Build history of the part. All positions in model axes, mm. A direction names the side the tool comes from. Coordinates: 2 decimals unless noted, no trailing zeros. Order: outer loops, then holes, each group sorted by start corner. A loop starts at its lowest first (then second) coordinate and runs counter-clockwise, first axis right, second up. Notation, with made-up numbers: (35, 53) - (72, 53) arc R8 ccw to (72, 58) - close; hole circle Ø3 at (89.25, 51). An arc over 180 degrees is marked (long way). Write each question's results on one line, items separated by ' | '.
from build123d import *

# Parameters (mm, degrees)
SKETCH1_R               = 13
SKETCH1_R_2             = 1.6
BOSS_EXTRUDE1_DEPTH     = 6.35
SKETCH2_W               = 5.8
SKETCH2_H               = 43
BOSS_EXTRUDE2_DEPTH     = 25.4
CUT_EXTRUDE1_DEPTH      = 26.4
CUT_EXTRUDE1_DEPTH_BACK = 7.35
SKETCH5_R               = 3.571875
CUT_EXTRUDE2_DEPTH      = 49.8
CUT_EXTRUDE2_DEPTH_BACK = 6.8
CHAMFER1_SIZE           = 5


with BuildPart() as part:
    # Sketch1 → Boss-Extrude1 (new body)
    with BuildSketch(Plane.XY):
        Polygon((-21.5, 21.5), (21.5, 21.5), (27.3, 21.5), (27.3, -21.5), (21.5, -21.5), (-21.5, -21.5), (-27.3, -21.5), (-27.3, 21.5), align=None)
        Circle(SKETCH1_R, mode=Mode.SUBTRACT)
        with Locations((-15.5, 15.5)):
            Circle(SKETCH1_R_2, mode=Mode.SUBTRACT)
        with Locations((15.5, 15.5)):
            Circle(SKETCH1_R_2, mode=Mode.SUBTRACT)
        with Locations((15.5, -15.5)):
            Circle(SKETCH1_R_2, mode=Mode.SUBTRACT)
        with Locations((-15.5, -15.5)):
            Circle(SKETCH1_R_2, mode=Mode.SUBTRACT)
    extrude(amount=BOSS_EXTRUDE1_DEPTH)

    # Sketch2 → Boss-Extrude2 (add)
    with BuildSketch(Plane.XY.offset(6.35)):
        with Locations((-24.4, 0)):
            Rectangle(SKETCH2_W, SKETCH2_H)
        with Locations((24.4, 0)):
            Rectangle(SKETCH2_W, SKETCH2_H)
    extrude(amount=BOSS_EXTRUDE2_DEPTH)

    # Sketch4 → Cut-Extrude1 (cut, two sides)
    with BuildSketch(Plane.XY.offset(6.35)) as cut_extrude1_sk:
        Polygon((-27.3, 12.7), (-21.5, 12.7), (-21.5, 16.5), (-16.5, 21.5), (-21.5, 21.5), (-27.3, 21.5), align=None)
        Polygon((21.5, 21.5), (16.5, 21.5), (21.5, 16.5), (21.5, 12.7), (27.3, 12.7), (27.3, 21.5), align=None)
        Polygon((27.3, -21.5), (27.3, -12.7), (21.5, -12.7), (21.5, -16.5), (16.5, -21.5), (21.5, -21.5), align=None)
        Polygon((-27.3, -21.5), (-21.5, -21.5), (-16.5, -21.5), (-21.5, -16.5), (-21.5, -12.7), (-27.3, -12.7), align=None)
    extrude(amount=CUT_EXTRUDE1_DEPTH, mode=Mode.SUBTRACT)
    extrude(cut_extrude1_sk.sketch, amount=-CUT_EXTRUDE1_DEPTH_BACK, mode=Mode.SUBTRACT)

    # Sketch5 → Cut-Extrude2 (cut, two sides)
    with BuildSketch(Plane(origin=(-21.5, 0, 0), x_dir=(0, 0, -1), z_dir=(1, 0, 0))) as cut_extrude2_sk:
        with Locations((-19.05, 0)):
            Circle(SKETCH5_R)
    extrude(amount=CUT_EXTRUDE2_DEPTH, mode=Mode.SUBTRACT)
    extrude(cut_extrude2_sk.sketch, amount=-CUT_EXTRUDE2_DEPTH_BACK, mode=Mode.SUBTRACT)

    # Chamfer1
    chamfer1_edges = [part.edges().sort_by_distance(p)[0] for p in [
        (21.5, -12.7, 19.05),
        (-21.5, 12.7, 19.05),
        (-21.5, -12.7, 19.05),
        (21.5, 12.7, 19.05),
    ]]
    chamfer(chamfer1_edges, length=CHAMFER1_SIZE)


solid = part.part
1. Band-saw the part on A-A on z = 19.05. Give the cut face in (x, y), then the cut area to 3 significant figures.
Solved:
outline: (-27.3, -12.7) - (-26.5, -12.7) - (-21.5, -7.7) - (-21.5, -3.57) - (-27.3, -3.57) - close; (-27.3, 3.57) - (-21.5, 3.57) - (-21.5, 7.7) - (-26.5, 12.7) - (-27.3, 12.7) - close; (21.5, -7.7) - (26.5, -12.7) - (27.3, -12.7) - (27.3, -3.57) - (21.5, -3.57) - close; (21.5, 3.57) - (27.3, 3.57) - (27.3, 12.7) - (26.5, 12.7) - (21.5, 7.7) - close | area: 162 mm2
2. Drop flat-ended pins along their axis: pin 1 Ø4 at (x, y) = (15.5, -15.5) entering from +Z; pin 2 Ø4.5 at (x, z) = (25.5, 21.5) entering from +Y; pin 3 Ø4.5 at (x, z) = (-23, 11) entering from -Y; pin 4 Ø2.5 at (x, y) = (-15.5, 15.5) entering from -Z. Give the stop position or say it passes through.
Solved:
pin 1: stops at z = 6.35 | pin 2: stops at y = 12.7 | pin 3: stops at y = -11.45 | pin 4: passes through
3. Two-plate mould, pull along Y, no slides. Class faces 1 (the face through (-19, 19, 3)), 2 (the face through (-16.68, 16.58, 3.13)), 3 (the face through (24, -10.2, 18.9)), 4 (the face through (-24, 0, 31.75)): +Y half, -Y half, draft (parallel to the pull), parting line (faces both ways), or undercut.
Solved:
face 1: +Y half | face 2: undercut | face 3: -Y half | face 4: draft
4. Tool access for faces 5 (the face through (21.5, -15, 3)), 6 (the face through (-27, -12.7, 9)), 7 (the face through (21.5, -4, 22)): list every direction of +Z, -Z, +X, -X, +Y, -Y with a clear straight run to the whole face (end or side of a thin tool).
Solved:
face 5: +Z, -Z, +X, -Y | face 6: +Z, -Z, -X, -Y | face 7: +Z, +Y, -Y
5. Band-saw the part on D-D on z = 11. Give the cut face in (x, y).
Solved:
outline: (-27.3, -12.7) - (-26.5, -12.7) - (-21.5, -7.7) - (-21.5, 7.7) - (-26.5, 12.7) - (-27.3, 12.7) - close; (21.5, -7.7) - (26.5, -12.7) - (27.3, -12.7) - (27.3, 12.7) - (26.5, 12.7) - (21.5, 7.7) - close
6. Band-saw the part on B-B on y = 0. Give the cut face in (x, z), then the cut area to 3 significant figures.
Solved:
outline: (-27.3, 0) - (-13, 0) - (-13, 6.35) - (-21.5, 6.35) - (-21.5, 15.48) - (-27.3, 15.48) - close; (-27.3, 22.62) - (-21.5, 22.62) - (-21.5, 31.75) - (-27.3, 31.75) - close; (13, 0) - (27.3, 0) - (27.3, 15.48) - (21.5, 15.48) - (21.5, 6.35) - (13, 6.35) - close; (21.5, 22.62) - (27.3, 22.62) - (27.3, 31.75) - (21.5, 31.75) - close | area: 393 mm2
7. Probe line 1 (Y direction, x = 15.5, z = 4.5); line 2 (X direction, y = 2, z = 23.5); line 3 (Y direction, x = 0, z = 1.75). List the from-to ranges inside material, lowest first.
Solved:
line 1: y = -21.5 to -17.1, -13.9 to 13.9, 17.1 to 21.5 | line 2: x = -27.3 to -21.5, 21.5 to 27.3 | line 3: y = -21.5 to -13, 13 to 21.5
8. Band-saw the part on C-C on x = -15.5. Give the cut face in (y, z).
Solved:
outline: (-21.5, 0) - (-17.1, 0) - (-17.1, 6.35) - (-21.5, 6.35) - close; (-13.9, 0) - (13.9, 0) - (13.9, 6.35) - (-13.9, 6.35) - close; (17.1, 0) - (21.5, 0) - (21.5, 6.35) - (17.1, 6.35) - close
